Autodesk Fusion 360 part; units mm, degrees
sketch "Sketch1" plane through (0, 0, 0) normal (0, 1, 0) x (1, 0, 0)
  line L0 (-17.5, 17.5) -> (17.5, 17.5)
  line L1 (17.5, 17.5) -> (17.5, -17.5)
  line L2 (17.5, -17.5) -> (-17.5, -17.5)
  line L3 (-17.5, -17.5) -> (-17.5, 17.5)
  line L4 (-17.5, 17.5) -> (17.5, -17.5) construction
  line L5 (17.5, 17.5) -> (-17.5, -17.5) construction
  dimension "d1" = 35
  dimension "d2" = 35
extrude "Extrude1" add sketch "Sketch1" along normal blind 50 makes body 1
sketch "Sketch2" plane through (0, 50, 0) normal (0, 1, 0) x (-1, 0, 0)
  line L0 (17.5, 17.5) -> (-17.5, 17.5)
  line L1 (-17.5, 17.5) -> (-17.5, -17.5)
  line L2 (-17.5, -17.5) -> (17.5, -17.5)
  line L3 (17.5, -17.5) -> (17.5, 17.5)
  circle A0 centre (0, 0) radius 5.05
  dimension "d5" = 10.1
extrude "Extrude2" cut sketch "Sketch2" against normal blind 20 contours A0 bodies 1
sketch "Sketch3" plane through (17.5, 0, 0) normal (1, 0, 0) x (0, 0, -1)
  line L0 (-17.5, 0) -> (17.5, 0)
  line L1 (17.5, 0) -> (17.5, 50)
  line L2 (17.5, 50) -> (-17.5, 50)
  line L3 (-17.5, 50) -> (-17.5, 0)
  line L4 (-10.5, 7) -> (10.5, 7)
  line L5 (10.5, 7) -> (10.5, 43)
  line L6 (10.5, 43) -> (-10.5, 43)
  line L7 (-10.5, 43) -> (-10.5, 7)
  line L8 (-5.05, 30) -> (5.05, 30)
  line L9 (-10.5, 7) -> (-10.5, 19) construction
  line L10 (-10.5, 19) -> (10.5, 19)
  dimension "d8" = -7
  dimension "d10" = 12
extrude "Extrude3" cut sketch "Sketch3" against normal blind 20 contours L4 L5 L7 L10 bodies 1
draft "Draft1" angle 45 neutral plane through (-2.5, 0, 0) pull (1, 0, 0) 1 faces at (10.8333, 19, 3.5) on bodies 1
fillet "Fillet2" radius 2 4 edges at (-17.5, 25, 17.5) (17.5, 25, 17.5) (17.5, 25, -17.5) (-17.5, 25, -17.5) on bodies 1
delete_face "DeleteFace2" 1 faces at (-2.5, 15, -3.5) on bodies 1
copy_body "Body->Comp1" bodies 1 removing the originals makes body 2 in component "Desk Mount"
component "Desk Mount" placed x (1, 0, 0) y (0, 1, 0) z (0, 0, 1) at (0, 0, 0)
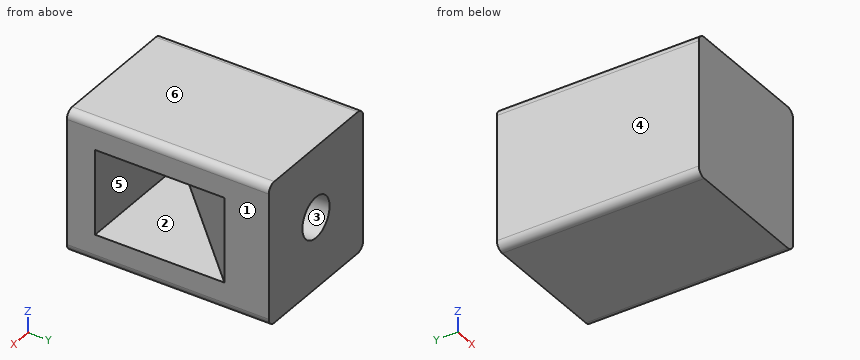
Input: part model. Units: mm. Frame: model coordinates. Face numbers are marked on the shaded views. A direction names the side the tool comes from. Round coordinates to 2 decimals unless told otherwise and drop trailing zeros. Order: outer loops, then holes, each group sorted by start corner. A loop starts at its lowest first (then second) coordinate and runs counter-clockwise, first axis right, second up. Notation, with made-up numbers: (-19.5, 48.25) - (-1.5, 48.25) arc R19 ccw to (-1.5, 53.25) - close; hole circle Ø4 at (58.5, 43). An arc over 180 degrees is marked (long way). Answer as a JSON object with one key per item and string values. Group by question number.
(1) Pin query (flat end, axial travel): P1, Ø5, axis at x = 0, z = -2, coming from the +Y side; P2, Ø8, axis at x = 0, z = 0, coming from the -Y side. Return the tip coordinate at first contact, or that it passes through.
(2) Material intervals for probe 1 along Z at (x, y) = (0, 36); probe 2 along Y at (x, z) = (10, -2); probe 3 along Y at (x, z) = (16.5, -9), sorted ascending. Write a range as from..to.
(3) Cut plane B-B (x = -10.5). Return loops of the section in (y, z).
(4) Reachability of the marked faces 1, 2 and 3 from +Z, -Z, +X, -X, +Y, -Y: full face, straight path, thin tool, end or side. Return the list, or none.
(5) Cut plane C-C (z = 0). Return loops of the section in (x, y).
(6) Draft query along Z for the marked faces 4, 5 and 6. Return one class per face: released by +Z, released by -Z, zero draft, split by the parting line, or undercut.
(7) Cut plane A-A (y = 35). Return loops of the section in (x, z).
(8) Cut plane D-D (y = 15.5). Return loops of the section in (x, z), then the cut area to 3 significant figures.
Here are the results:
{
 "1": {"P1": "stops at y = 30", "P2": "stops at y = 0"},
 "2": {"probe 1": "z = -17.5..-5.05, 5.05..17.5", "probe 2": "y = 0..7, 31.5..50", "probe 3": "y = 0..7, 38..50"},
 "3": {"outline": "(0, -17.5) - (50, -17.5) - (50, 17.5) - (0, 17.5) - close; hole (7, -10.5) - (11, -10.5) - (11, 10.5) - (7, 10.5) - close"},
 "4": {"face 1": "+Z, -Z, +X, +Y, -Y", "face 2": "+X", "face 3": "+Y"},
 "5": {"outline": "(-17.5, 0) - (17.5, 0) - (17.5, 7) - (-14.5, 7) - (17.5, 39) - (17.5, 50) - (5.05, 50) - (5.05, 30) - (-5.05, 30) - (-5.05, 50) - (-17.5, 50) - close"},
 "6": {"face 4": "zero draft", "face 5": "undercut", "face 6": "released by +Z"},
 "7": {"outline": "(-17.5, -15.5) arc R2 ccw to (-15.5, -17.5) - (15.5, -17.5) arc R2 ccw to (17.5, -15.5) - (17.5, -10.5) - (13.5, -10.5) - (13.5, 10.5) - (17.5, 10.5) - (17.5, 15.5) arc R2 ccw to (15.5, 17.5) - (-15.5, 17.5) arc R2 ccw to (-17.5, 15.5) - close; hole circle Ø10.1 at (0, 0)"},
 "8": {"outline": "(-17.5, -15.5) arc R2 ccw to (-15.5, -17.5) - (15.5, -17.5) arc R2 ccw to (17.5, -15.5) - (17.5, -10.5) - (-6, -10.5) - (-6, 10.5) - (17.5, 10.5) - (17.5, 15.5) arc R2 ccw to (15.5, 17.5) - (-15.5, 17.5) arc R2 ccw to (-17.5, 15.5) - close", "area": "728 mm^2"}
}
